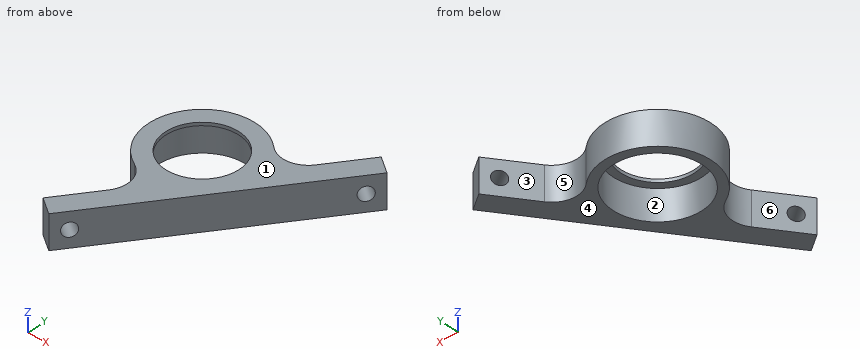
Autodesk Inventor part; units mm, degrees
ref_plane "YZ Plane" through (0, 0, 0) normal (1, 0, 0) x (0, 1, 0)
ref_plane "XZ Plane" through (0, 0, 0) normal (0, 1, 0) x (-1, 0, 0)
ref_plane "XY Plane" through (0, 0, 0) normal (0, 0, 1) x (1, 0, 0)
sketch "Sketch1" plane through (0, 0, 0) normal (0, 0, 1) x (1, 0, 0)
  circle A0 centre (0, 0) radius 11
  arc A1 (9.103, 9.9692) -> (-6.4691, -11.8491) centre (0, 0) ccw
  line L0 (122.2578, 146.7857) -> (-99.0763, -163.3307)
  arc A2 (9.103, 9.9692) -> (18.8408, 11) centre (13.515, 14.8011) ccw
  line L1 (18.8408, 11) -> (26.1613, 21.2569)
  line L2 (26.1613, 21.2569) -> (30.471, 18.181)
  line L3 (0, 0) -> (9.5455, -6.8127)
  line L4 (-7.2894, -34.726) -> (30.471, 18.181)
  arc A3 (-4.2786, -21.3932) -> (-6.4691, -11.8491) centre (-9.6045, -17.5921) ccw
  line L5 (-4.2786, -21.3932) -> (-11.5991, -31.6501)
  line L6 (-11.5991, -31.6501) -> (-7.2894, -34.726)
  line L7 (-7.2894, -34.726) -> (30.471, 18.181)
  circle A4 centre (0, 0) radius 11.25
  point P0 (0, 0)
  point P1 (-99.0763, -163.3307)
  point P2 (122.2578, 146.7857)
  dimension "d0" = 2.5
  dimension "d12" = 65
  dimension "d15" = 22.5
extrude "Extrusion1" add sketch "Sketch1" along normal blind 8.5 contours A2 L1 L2 L0 L6 L5 A3 A1
sketch "Sketch2" plane through (0, 0, 8.5) normal (0, 0, 1) x (1, 0, 0)
  circle A0 centre (0, 0) radius 9.2831
  circle A1 centre (0, 0) radius 10.96
  circle A2 centre (0, 0) radius 13.5
  dimension "d3" = 18.5661
extrude "Extrusion2" add sketch "Sketch2" against normal blind 0.8 contours A1 | A2
sketch "Sketch3" plane through (-11.5991, -31.6501, 0) normal (-0.8139539, 0.5809295, 0) x (0, 0, 1)
  line L0 (0, 12.6013) -> (0, 0)
  line L1 (0, 0) -> (8.5, 0)
  line L2 (8.5, 12.6013) -> (8.5, 0)
  line L3 (0, 12.6013) -> (8.5, 12.6013)
  line L4 (0, 65) -> (0, 52.3987)
  line L5 (0, 52.3987) -> (8.5, 52.3987)
  line L6 (8.5, 65) -> (8.5, 52.3987)
  line L7 (0, 65) -> (8.5, 65)
  line L8 (3.4344, 32.2582) -> (4.7482, 32.2582)
  circle A0 centre (4.25, 4) radius 1.75
  circle A1 centre (4.25, 61) radius 1.75
  point P0 (0, 32.5)
  dimension "d10" = 3.5
  dimension "d11" = 3.5
  dimension "d13" = 4
  dimension "d14" = 4
extrude "Extrusion3" cut sketch "Sketch3" against normal up to surface (5.2948 mm away) contours A0 | A1
properties part number "bearing block"
Design review of the part built by this model. Coordinates are the model's own, in mm. Face numbers are marked on the shaded views. A direction names the side the tool comes from. Coordinates: 2 decimals unless noted, no trailing zeros. Order: outer loops, then holes, each group sorted by start corner. A loop starts at its lowest first (then second) coordinate and runs counter-clockwise, first axis right, second up.
Item 1: The part is to be moulded in two halves that separate along X. For the marked faces 4, 5 and 6, say which applies: pulls with the +X half, pulls with the -X half, needs draft (parallel to the pull), parting line crosses it, or undercut.
Item 2: For pin 1 Ø3 at (x, z) = (21.5, 3.5) entering from -Y; pin 2 Ø3 at (y, z) = (13, 7.5) entering from +X; pin 3 Ø1.5 at (y, z) = (-20.5, 1.5) entering from +X, all flat-tipped, find the tip position at first contact; note any pin that passes through.
Item 3: Take a section at A-A, the plane y = -1. Write out the cut boundary in (x, z), then the cut area to 3 significant figures.
Item 4: Take a section at B-B, the plane z = 4.25. Write out the cut boundary in (x, y), then the cut area to 3 significant figures.
Item 5: For line 1 (X direction, y = 2.5, z = 5.5); line 2 (Y direction, x = -1, z = 1); line 3 (Y direction, x = 0, z = 2), list the stretches that pass through material, from the lowest coordinate up.
Item 6: Take a section at C-C, the plane x = 0. Write out the cut boundary in (y, z).
Item 7: Take a section at D-D, the plane y = -10. Write out the cut boundary in (x, z), then the cut area to 3 significant figures.
Item 8: For the marked faces 1, 2 and 3, list the 3-axis set-ups (+Z, -Z, +X, -X, +Y, -Y) from which the entire face can be reached by the end or side of a thin tool; tool diameter is ignored.
The answers:
1. face 4: needs draft
1. face 5: undercut
1. face 6: pulls with the -X half
2. pin 1: stops at y = 3.51
2. pin 2: stops at x = 27.84
2. pin 3: stops at x = 3.4
3. outline: (-13.46, 0) - (-11.21, 0) - (-11.21, 7.7) - (-9.23, 7.7) - (-9.23, 8.5) - (-13.46, 8.5) - close; (9.23, 7.7) - (11.21, 7.7) - (11.21, 0) - (16.78, 0) - (16.78, 8.5) - (9.23, 8.5) - close
3. area: 69.7 mm2
4. outline: (-11.6, -31.65) - (-7.29, -34.73) - (-5.98, -32.89) - (-10.29, -29.82) - close; (-8.26, -26.97) - (-3.95, -30.05) - (27.13, 13.5) - (22.82, 16.58) - (18.84, 11) arc R6.54 cw to (9.1, 9.97) arc R13.5 ccw (long way) to (-6.47, -11.85) arc R6.54 cw to (-4.28, -21.39) - close; (24.85, 19.43) - (29.16, 16.35) - (30.47, 18.18) - (26.16, 21.26) - close; hole circle Ø22.5 at (0, 0)
4. area: 453 mm2
5. line 1: x = -13.27 to -10.97, 10.97 to 19.28
5. line 2: y = -25.91 to -11.21, 11.21 to 13.46
5. line 3: y = -24.51 to -11.25, 11.25 to 13.5
6. outline: (-24.51, 0) - (-11.25, 0) - (-11.25, 7.7) - (-9.28, 7.7) - (-9.28, 8.5) - (-24.51, 8.5) - close; (9.28, 7.7) - (11.25, 7.7) - (11.25, 0) - (13.5, 0) - (13.5, 8.5) - (9.28, 8.5) - close
7. outline: (-9.07, 0) - (-5.15, 0) - (-5.15, 7.7) - (5.15, 7.7) - (5.15, 0) - (10.36, 0) - (10.36, 8.5) - (-9.07, 8.5) - close
7. area: 85.8 mm2
8. face 1: +Z, +X, -X, +Y, -Y
8. face 2: -Z
8. face 3: +Z, -Z, +Y
